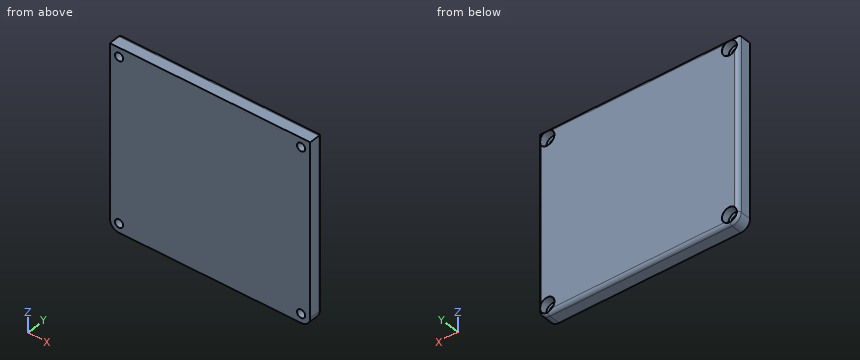
```python
from build123d import *

# Parameters (mm, degrees)
SKETCH2_W                                    = 110
SKETCH2_H                                    = 100
BOSS_EXTRUDE1_DEPTH                          = 8
FILLET2_R                                    = 2
FILLET3_R                                    = 5
CBORE_FOR_M4_HEX_SOCKET_HEAD_CAP_SCR_2_COUNT = 2
CBORE_FOR_M4_HEX_SOCKET_HEAD_CAP_SCR_2_PITCH = 100
CBORE_FOR_M4_HEX_SOCKET_HEAD_CAP_SCR_3_COUNT = 2
CBORE_FOR_M4_HEX_SOCKET_HEAD_CAP_SCR_3_PITCH = 134.536240471
CBORE_FOR_M4_HEX_SOCKET_HEAD_CAP_SCR_4_COUNT = 2
CBORE_FOR_M4_HEX_SOCKET_HEAD_CAP_SCR_4_PITCH = 90


with BuildPart() as part:
    # Sketch2 → Boss-Extrude1 (new body)
    with BuildSketch(Plane(origin=(0, 0, 0), x_dir=(1, 0, 0), z_dir=(0, 1, 0))):
        Rectangle(SKETCH2_W, SKETCH2_H)
    extrude(amount=BOSS_EXTRUDE1_DEPTH)

    # Fillet2
    fillet2_edges = [part.edges().sort_by_distance(p)[0] for p in [
        (-55, 8, 0),
        (0, 8, 50),
        (55, 8, 0),
        (0, 8, -50),
    ]]
    fillet(fillet2_edges, radius=FILLET2_R)

    # Fillet3
    # the kernel refuses this fillet: 5 mm, written as the material it takes off along each edge
    with BuildSketch(Plane(origin=(-50, 8, -45), x_dir=(0, 0, -1), z_dir=(1, 0, 0))) as fillet3_piece_1:
        with BuildLine():
            CenterArc((3, -2), 2, 0, 90)
            Line((5, -2), (5, 0))
            Line((5, 0), (3, 0))
        make_face()
    revolve(axis=Axis((-50, 8, -45), (0, 1, 0)), revolution_arc=90, mode=Mode.SUBTRACT)
    with BuildSketch(Plane(origin=(50, 8, -45), x_dir=(1, 0, 0), z_dir=(0, 0, 1))) as fillet3_piece_2:
        with BuildLine():
            CenterArc((3, -2), 2, 0, 90)
            Line((5, -2), (5, 0))
            Line((5, 0), (3, 0))
        make_face()
    revolve(axis=Axis((50, 8, -45), (0, 1, 0)), revolution_arc=90, mode=Mode.SUBTRACT)
    with BuildSketch(Plane(origin=(-55, -12.5, -50), x_dir=(1, 0, 0), z_dir=(0, 1, 0))) as fillet3_piece_3:
        with BuildLine():
            CenterArc((FILLET3_R, -FILLET3_R), FILLET3_R, 90, 90)
            Line((0, -FILLET3_R), (0, 0))
            Line((0, 0), (FILLET3_R, 0))
        make_face()
    extrude(amount=20.5, mode=Mode.SUBTRACT)
    with BuildSketch(Plane(origin=(55, -12.5, -50), x_dir=(-1, 0, 0), z_dir=(0, 1, 0))) as fillet3_piece_4:
        with BuildLine():
            CenterArc((FILLET3_R, FILLET3_R), FILLET3_R, 180, 90)
            Line((0, FILLET3_R), (0, 0))
            Line((0, 0), (FILLET3_R, 0))
        make_face()
    extrude(amount=20.5, mode=Mode.SUBTRACT)

    # Sketch4 → CBORE for M4 Hex Socket Head Cap Screw1 (revolve, cut)
    with BuildSketch(Plane(origin=(50, 8, -45), x_dir=(0, 0, 1), z_dir=(1, 0, 0))):
        Polygon((0, 0), (0, 11.451936393), (2.25, 10.1), (2.25, 4.4), (4, 4.4), (4, 0.025), (4.025, 0), align=None)
    cbore_for_m4_hex_socket_head_cap_screw1 = revolve(axis=Axis((50, 14.35, -45), (0, -1, 0)), mode=Mode.SUBTRACT)

    # CBORE for M4 Hex Socket Head Cap Scr 2: CBORE for M4 Hex Socket Head Cap Screw1 ×2
    with Locations(*[(-i * CBORE_FOR_M4_HEX_SOCKET_HEAD_CAP_SCR_2_PITCH, 0, 0) for i in range(1, CBORE_FOR_M4_HEX_SOCKET_HEAD_CAP_SCR_2_COUNT)]):
        add(cbore_for_m4_hex_socket_head_cap_screw1, mode=Mode.SUBTRACT)

    # CBORE for M4 Hex Socket Head Cap Scr 3: CBORE for M4 Hex Socket Head Cap Screw1 ×2
    with Locations(*[Vector(-0.7432941462471664, 0, 0.6689647316224497) * (i * CBORE_FOR_M4_HEX_SOCKET_HEAD_CAP_SCR_3_PITCH) for i in range(1, CBORE_FOR_M4_HEX_SOCKET_HEAD_CAP_SCR_3_COUNT)]):
        add(cbore_for_m4_hex_socket_head_cap_screw1, mode=Mode.SUBTRACT)

    # CBORE for M4 Hex Socket Head Cap Scr 4: CBORE for M4 Hex Socket Head Cap Screw1 ×2
    with Locations(*[(0, 0, i * CBORE_FOR_M4_HEX_SOCKET_HEAD_CAP_SCR_4_PITCH) for i in range(1, CBORE_FOR_M4_HEX_SOCKET_HEAD_CAP_SCR_4_COUNT)]):
        add(cbore_for_m4_hex_socket_head_cap_screw1, mode=Mode.SUBTRACT)


solid = part.part
```
Geometry: final body of the model. Coordinates: model frame, mm. Round coordinates to 2 decimals unless told otherwise and drop trailing zeros. Write each loop counter-clockwise with the first axis right and the second up, starting at its lowest first coordinate (ties: lowest second). Pieces come first, ordered by that corner, then holes. Notation, with made-up numbers: M -31.75,67.5 L -7.75,67.5 A21 ccw -7.75,89.5 Z; hole C -33,-2.5 d7. An arc over 180 degrees is marked long. Answer in a Markdown table with one row per item. Add a question column.
(1) Cut plane A-A, the plane z = 45. Return the cut outline in (x, y) (3 decimals), then the cut area to 3 significant figures.
(2) Ray query, L1, parallel to X at y = 1.45, z = 45; L2, parallel to Z at x = -50, y = 5.8; L3, parallel to X at y = 5.2, z = 45. Return the intervals inside material, ascending.
(3) Contact query for flat-ended pins moving along their axis: pin 1 (2 mm diameter, centred on x = -33.5, z = -4.5, fed in from -Y); pin 2 (2.5 mm diameter, centred on x = -50, z = 45, fed in from -Y); pin 3 (4 mm diameter, centred on x = -49.5, z = -46.5, fed in from +Y); pin 4 (4 mm diameter, centred on x = 51.5, z = -47, fed in from +Y). Output: stop coordinate, or through.
Established:
| question | item | result |
|---|---|---|
| 1 | outline | M -55,0 L -52.25,0 L -52.25,3.6 L -54,3.6 L -54,7.732 A2 ccw -55,6 Z; M -47.75,0 L 47.75,0 L 47.75,3.6 L 46,3.6 L 46,7.975 L 45.975,8 L -45.975,8 L -46,7.975 L -46,3.6 L -47.75,3.6 Z; M 52.25,0 L 55,0 L 55,6 A2 ccw 54,7.732 L 54,3.6 L 52.25,3.6 Z |
| 1 | area | 776 mm² |
| 2 | L1 | -55 to -52.25, -47.75 to 47.75, 52.25 to 55 |
| 2 | L2 | -50 to -49, -41 to 41, 49 to 50 |
| 2 | L3 | -55 to -54, -46 to 46, 54 to 55 |
| 3 | pin 1 | y = 0 |
| 3 | pin 2 | through |
| 3 | pin 3 | y = 3.6 |
| 3 | pin 4 | y = 7.73 |
